Input: part model. Units: mm. Frame: model coordinates. Give positions to 0.01 mm unless a question says otherwise; leave off trailing zeros. Loops run counter-clockwise (first coordinate to the right, second up) from the corner with the lowest first, then second, coordinate; pieces in that order, holes last. Notation, with made-up numbers: M 21,-9.75 L 42,-9.75 A21 cw 42,1.25 Z; hole C 8,34.5 d7. An arc over 180 degrees is marked long. Answer as a JSON object with one key per item and string values. Group by question number.
1) Section query A-A on x = -51. Return loops of the section in (y, z), plus the area to 3 significant figures.
2) Section query B-B on y = -2. Return loops of the section in (x, z).
3) Section query D-D on y = -34. Return loops of the section in (x, z).
4) Ray query, L1, parallel to Y at x = -47, z = 2.25; L2, parallel to Y at x = -42, z = 4.7; L3, parallel to Y at x = -40, z = 0.45. Return the intervals inside material, ascending.
5) First-contact query: P1, Ø1, axis at y = -40.5, z = 3, coming from the +X side; P2, Ø2, axis at x = -42, z = 3, coming from the +Y side; P3, Ø1, axis at x = -49.5, z = 4.5, coming from the -Y side. Flat tips, straight axial feed; report the tip coordinate or a pass-through.
6) Section query C-C on z = 3.65. Return loops of the section in (x, y) (1 decimal).
Autodesk Inventor part; units mm, degrees
ref_plane "YZ Plane" through (0, 0, 0) normal (1, 0, 0) x (0, 1, 0)
ref_plane "XZ Plane" through (0, 0, 0) normal (0, 1, 0) x (-1, 0, 0)
ref_plane "XY Plane" through (0, 0, 0) normal (0, 0, 1) x (1, 0, 0)
sketch "Sketch1" plane through (0, 0, 0) normal (0, 0, 1) x (1, 0, 0)
  arc A0 (-46.1263, 10.632) -> (-62.6331, -17.4708) centre (15.0732, -44.2142) ccw
  arc A1 (-62.6331, -17.4708) -> (-54.2395, -22.9066) centre (-57.7619, -19.1473) ccw
  arc A2 (-33.338, 11.3144) -> (-54.2395, -22.9066) centre (22.5624, -46.3221) ccw
  arc A3 (-33.338, 11.3144) -> (-46.1263, 10.632) centre (-39.3918, 4.5967) ccw construction
  arc A4 (-62.8989, -19.5348) -> (-54.0515, -50.903) centre (19.0478, -13.3535) ccw
  arc A5 (-54.0515, -50.903) -> (-41.8534, -54.8035) centre (-46.0076, -46.7711) ccw
  arc A6 (-53.4019, -16.4032) -> (-41.8534, -54.8035) centre (26.8267, -13.212) ccw
  arc A7 (-53.4019, -16.4032) -> (-62.8989, -19.5348) centre (-57.7619, -19.1473) ccw
  arc A8 (-29.559, -59.3436) -> (2.6139, -54.1332) centre (-26.3493, 22.7733) ccw
  arc A9 (2.6139, -54.1332) -> (1.4472, -44.2015) centre (0.7983, -49.3121) ccw
  arc A10 (-38.241, -49.9292) -> (1.4472, -44.2015) centre (-29.5023, 29.8859) ccw
  arc A11 (-38.241, -49.9292) -> (-29.559, -59.3436) centre (-29.2058, -50.3074) ccw
  arc A12 (4.4376, -52.9584) -> (22.4821, -25.8173) centre (-53.6163, 5.2072) ccw
  arc A13 (22.4821, -25.8173) -> (17.499, -14.02) centre (14.1082, -22.4033) ccw
  arc A14 (-4.1234, -47.7902) -> (17.499, -14.02) centre (-58.7892, 11.0185) ccw
  arc A15 (-4.1234, -47.7902) -> (4.4376, -52.9584) centre (0.7983, -49.3121) ccw
  arc A16 (-44.7504, -1.2652) -> (-41.8534, -54.8035) centre (-4.8947, -25.9562) ccw
  arc A17 (-46.1263, 10.632) -> (-62.6331, -17.4708) centre (15.0732, -44.2142) ccw
  arc A18 (-62.6331, -17.4708) -> (-54.0515, -50.903) centre (13.2398, -15.8127) ccw
  arc A19 (-54.0515, -50.903) -> (-41.8534, -54.8035) centre (-46.0076, -46.7711) ccw
  circle A20 centre (-40.1686, 5.2928) radius 8
  arc A21 (-44.7504, -1.2652) -> (-41.8534, -54.8035) centre (-4.8947, -25.9562) ccw
  arc A22 (-46.1263, 10.632) -> (-44.7504, -1.2652) centre (-40.1686, 5.2928) ccw
  point P0 (0, 0)
  dimension "d4" = 16
extrude "Extrusion3" add sketch "Sketch1" along normal blind 5.5 contours A20 A16 A2 A6 A7 A0 | A20 A2 | A7 A6 A2 A1 A18 | A20 A2 | A1 A2 A6 A16 A5 A4 A18 | A16 A6 A2 | A4 A18
properties part number "BHENCHOD FINGER"
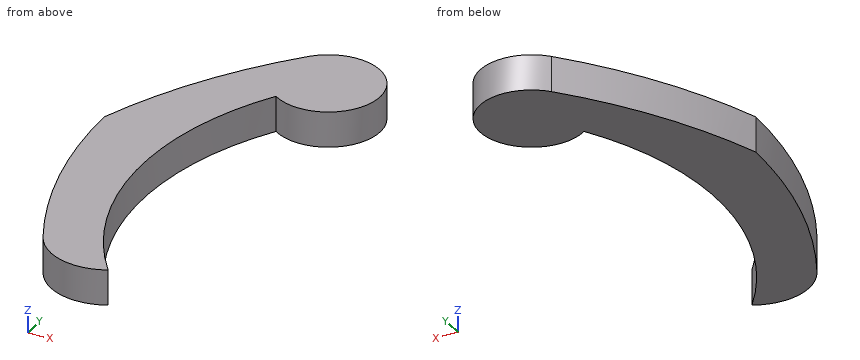
Output:
{
 "1": {"outline": "M -54.31,0 L -34.47,0 L -34.47,5.5 L -54.31,5.5 Z; M -17.45,0 L 4.65,0 L 4.65,5.5 L -17.45,5.5 Z", "area": "231 mm^2"},
 "2": {"outline": "M -55.44,0 L -45.2,0 L -45.2,5.5 L -55.44,5.5 Z; M -43.46,0 L -36.88,0 L -36.88,5.5 L -43.46,5.5 Z"},
 "3": {"outline": "M -60.44,0 L -51.08,0 L -51.08,5.5 L -60.44,5.5 Z"},
 "4": {"L1": "y = -55.76 to -46.58, -5.33 to 9.64", "L2": "y = -54.88 to -54.61, -2.49 to 13.08", "L3": "y = -2.71 to 13.29"},
 "5": {"P1": "stops at x = -49.3", "P2": "stops at y = 13.25", "P3": "stops at y = -55.3"},
 "6": {"outline": "M -62.6,-17.5 A75.9 ccw -54.1,-50.9 A9 ccw -41.9,-54.8 A46.9 cw -44.8,-1.3 A8 ccw long -46.1,10.6 A82.2 ccw Z"}
}
